Here's how the part is built. I have some questions about the finished solid (model axes, mm). Face numbers are marked on the shaded views. A direction names the side the tool comes from. Coordinates: 2 decimals unless noted, no trailing zeros. Write each loop counter-clockwise with the first axis right and the second up, starting at its lowest first coordinate (ties: lowest second). Pieces come first, ordered by that corner, then holes. Notation, with made-up numbers: (30.5, 16.5) -> (56.5, 16.5) arc R20 ccw to (56.5, 31.5) -> close; hole circle Ø9 at (83.25, 85). An arc over 180 degrees is marked (long way). Use a Markdown table: item, result. Add a question column.
Autodesk Inventor part; units mm, degrees
ref_plane "Work Plane1" through (30.1625, 0, 0) normal (0, 0, -1) x (1, 0, 0)
ref_plane "YZ Plane" through (0, 0, 0) normal (1, 0, 0) x (0, 1, 0)
ref_plane "XZ Plane" through (0, 0, 0) normal (0, 1, 0) x (-1, 0, 0)
sketch "Sketch1" plane through (0, 0, 0) normal (0, 0, 1) x (1, 0, 0)
  line L0 (-1.8, 0) -> (20, 0)
  line L1 (20, 0) -> (20, 1.5)
  line L2 (20, 1.5) -> (1, 1.5)
  line L3 (1, 1.5) -> (0.6932, 1.1935)
  line L4 (0.6932, 1.1935) -> (0, 1.1935)
  line L5 (0, 1.1935) -> (0, 3)
  line L6 (-6.16, 0) -> (24.36, 0)
  line L7 (0, -0.6) -> (0, 3.6)
  line L8 (-1.8, 0) -> (-1.8, 2.9997)
  line L9 (0, 3) -> (-1.8, 2.9997)
  line L10 (1, 1.5) -> (0, 1.5) construction
  dimension "d0" = 20
  dimension "d1" = 19
  dimension "d2" = 0.3068
  dimension "d3" = 1.8
  dimension "d4" = 3
  dimension "d5" = 2.387
  dimension "d9" = 6
  dimension "d10" = 0.01
revolve "Body" add sketch "Sketch1" angle 360 about axis through (-1.8, 0, 0) along (1, 0, 0)
sketch "Sketch2" plane through (-1.8, 0, 0) normal (-1, 0, 0) x (0, 0, 1)
  circle A0 centre (0, 0) radius 3
  line L0 (0, 0) -> (0, 2.9997)
  line L1 (-3, 0.5) -> (3, 0.5)
  line L2 (3, 0.5) -> (3, -0.5)
  line L3 (3, -0.5) -> (-3, -0.5)
  line L4 (-3, -0.5) -> (-3, 0.5)
  line L5 (-3, 0) -> (3, 0) construction
  line L6 (0, 0.5) -> (0, -0.5) construction
  dimension "d11" = 1
  dimension "d12" = 6
fillet "Fillet1" radius 1.2 1 edges at (-1.8, -2.9997, 0)
extrude "Slot" cut sketch "Sketch2" against normal blind 0.72 contours A0 L3 L1 | L2 L3 A0 | A0 L1 L2 | L3 L4 A0 | A0 L4 L1
thread "Thread"
chamfer "Chamfer1" distance 0.3067 distance2 0.3068 1 edges at (20, -1.5, 0) measured on face at (20, 0.3743, -0.3316)
ref_plane "Work Plane1" through (30.1625, 0, 0) normal (0, 0, -1) x (1, 0, 0)
equation "\"d11\" = SBR"
equation "\"d12\" = KOD"
equation "\"d14\" = RR"
equation "\"d19\" = STI"
equation "\"d15\" = GEL"
equation "\"d17\" = -0.5 * SPD + 0.5 * GD"
equation "\"d0\" = NLG"
equation "\"d1\" = GEL"
equation "\"d3\" = KOH"
equation "\"d4\" = GD"
equation "\"d5\" = BDM"
equation "\"d9\" = KOD"
equation "\"d10\" = KEWI"
equation "\"GD\" = NND"
equation "\"NLG\" = 20"
equation "\"GEL\" = 19"
equation "\"KOD\" = 6"
equation "\"KOH\" = 1.8"
equation "\"GAL\" = 0.61345 * PTC"
equation "\"SPD\" = NND - 1.2269 * PTC"
equation "\"BDM\" = 2.387"
equation "\"GUL\" = 0.61345 * PTC"
equation "\"RR\" = 1.2"
equation "\"SBR\" = 1"
equation "\"STI\" = 0.72"
equation "\"KEWI\" = 0.01deg"
equation "\"PTC\" = 0.5"
equation "\"THREADDIA\" = 3"
equation "\"TOA\" = 30deg"
equation "\"NND\" = 3"
equation "\"RR1\" = 0.3"
equation "\"GD1\" = THREADDIA - 1.2269 * PTC"
properties part number "AS 1427 - M3 x 20(6)" material "Steel, Mild"
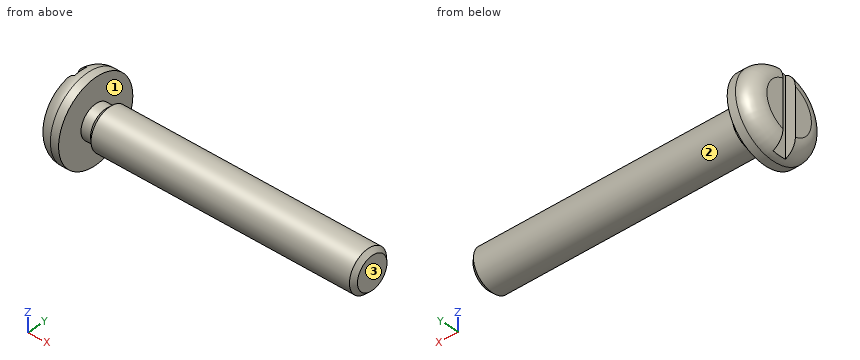
Q1. Please list where these lines run through material, in increasing order: line 1 (X direction, y = -1.5, z = 0.5); line 2 (X direction, y = 0, z = 1.75); line 3 (Z direction, x = 17.25, y = -0.75).
Q2. Suppose I cut it at C-C, the plane x = 17.25. Write out the boundary of the cut face in (y, z), and give its area (3 significant figures).
Q3. Suppose I cut it at A-A, the plane y = 0. Write out the boundary of the cut face in (x, z).
Q4. Suppose I cut it at B-B, the plane z = 0. Write out the boundary of the cut face in (x, y), and give its area (3 significant figures).
Q5. Which directions (+Z, -Z, +X, -X, +Y, -Y) give clear straight access to the entire face, cutting with the end or side of a thin tool? Please do the marked faces 1, 2 and 3.
Q6. Will these pins go through, and if not, where does the flat tip stop? pin 1 (1 mm diameter, centred on y = -2.5, z = 1, fed in from -X); pin 2 (0.6 mm diameter, centred on x = -1.5, z = -0.5, fed in from +Y); pin 3 (2 mm diameter, centred on x = 10, y = -1.5, fed in from -Z).
Answer key:
| question | item | result |
|---|---|---|
| 1 | line 1 | x = -1.8 to 0 |
| 1 | line 2 | x = -1.08 to 0 |
| 1 | line 3 | z = -1.3 to 1.3 |
| 2 | outline | circle Ø3 at (0, 0) |
| 2 | area | 7.07 mm^2 |
| 3 | outline | (-1.08, -2.9) arc R1.2 ccw to (-0.6, -3) -> (0, -3) -> (0, -1.19) -> (0.69, -1.19) -> (1, -1.5) -> (19.69, -1.5) -> (20, -1.19) -> (20, 1.19) -> (19.69, 1.5) -> (1, 1.5) -> (0.69, 1.19) -> (0, 1.19) -> (0, 3) -> (-0.6, 3) arc R1.2 ccw to (-1.08, 2.9) -> close |
| 4 | outline | (-1.8, -1.8) arc R1.2 ccw to (-0.6, -3) -> (0, -3) -> (0, -1.19) -> (0.69, -1.19) -> (1, -1.5) -> (19.69, -1.5) -> (20, -1.19) -> (20, 1.19) -> (19.69, 1.5) -> (1, 1.5) -> (0.69, 1.19) -> (0, 1.19) -> (0, 3) -> (-0.6, 3) arc R1.2 ccw to (-1.8, 1.8) -> (-1.8, 0.5) -> (-1.08, 0.5) -> (-1.08, -0.5) -> (-1.8, -0.5) -> close |
| 4 | area | 68.8 mm^2 |
| 5 | face 1 | none |
| 5 | face 2 | +X |
| 5 | face 3 | +Z, -Z, +X, +Y, -Y |
| 6 | pin 1 | stops at x = -1.73 |
| 6 | pin 2 | stops at y = 2.8 |
| 6 | pin 3 | stops at z = -1.41 |
